Model file for the job. Use its own axes, mm. A direction names the side the tool comes from. Round coordinates to 2 decimals unless told otherwise and drop trailing zeros. Order: outer loops, then holes, each group sorted by start corner. A loop starts at its lowest first (then second) coordinate and runs counter-clockwise, first axis right, second up. Notation, with made-up numbers: M 5.5,-21 L 27.5,-21 A17 ccw 27.5,5 Z; hole C 30,74.25 d5. An arc over 180 degrees is marked long. Return JSON: item names as keys, results as strings. Group by question number.
Item 1: Which spindle directions (+Z, -Z, +X, -X, +Y, -Y) get a long thin tool onto all of the face, cutting with end or side? Do faces 5 (the face through (64, 20, 0.711)), 6 (the face through (51, 17, 0)), 7 (the face through (19, 31, 4.369)). Say none if no direction does.
Item 2: Slice it at A-A on z = 2.3. Write the cut outline in (x, y), then the cut area to 3 significant figures.
Item 3: Probe line 1 along X through (y, z) = (31.5, 3.4); line 2 along Z through (x, y) = (23, 29); line 3 along Y through (x, z) = (10, 3.25). List the from-to ranges inside material, lowest first.
Item 4: Pin check, flat tip, straight feed: pin 1 Ø4.5 at (x, y) = (64, 20.5) entering from -Z. Stop position of the tip, or through.
Item 5: Slice it at B-B on x = 65. Write the cut outline in (y, z), then the cut area to 3 significant figures.
Item 6: Pull direction X, two halves, no side cores. Call faces 1 (the face through (51, 0, 3)), 2 (the face through (18.53, 27.89, 2.15)), 3 (the face through (104.14, 16, 3)), 4 (the face through (61.53, 20.27, 0.35)): pulls with the +X half, pulls with the -X half, needs draft (parallel to the pull), parting line crosses it, or undercut.
Item 7: Slice it at C-C on x = 28.5. Write the cut outline in (y, z), then the cut area to 3 significant figures.
from build123d import *

# Parameters (mm, degrees)
SKETCH1_W           = 104.14
SKETCH1_H           = 33.02
BOSS_EXTRUDE1_DEPTH = 5.334
CAVITY1_DEPTH       = 4.3688
CAVITY1_2_OUTLINE_R = 2.794
CAVITY1_2_DEPTH     = 0.7112


# Read off the part's stored shape, not the designer's step: Cavity1
with BuildPart() as part:
    # Sketch1 → Boss-Extrude1 (new body)
    with BuildSketch(Plane.XY):
        with Locations((52.07, 16.51)):
            Rectangle(SKETCH1_W, SKETCH1_H)
    extrude(amount=BOSS_EXTRUDE1_DEPTH)

    # Cavity1 outline → Cavity1 (cut)
    with BuildSketch(Plane.XY):
        with BuildLine():
            ThreePointArc((7.993160963, 33.02), (18.702187299, 27.889223026), (29.411213634, 33.02))
            Line((29.411213634, 33.02), (7.993160963, 33.02))
        make_face()
    extrude(amount=CAVITY1_DEPTH, mode=Mode.SUBTRACT)

    # Cavity1 2 outline → Cavity1 2 (cut)
    with BuildSketch(Plane.XY):
        with Locations((64.319453414, 20.142181246)):
            Circle(CAVITY1_2_OUTLINE_R)
    extrude(amount=CAVITY1_2_DEPTH, mode=Mode.SUBTRACT)


solid = part.part
Output values:
{
 "1": {"face 5": "-Z", "face 6": "-Z, +X, -X, +Y, -Y", "face 7": "-Z, +Y"},
 "2": {"outline": "M 0,0 L 104.14,0 L 104.14,33.02 L 29.41,33.02 A13.74 cw 7.99,33.02 L 0,33.02 Z", "area": "3,360 mm²"},
 "3": {"line 1": "0 to 9.42, 27.99 to 104.14", "line 2": "4.37 to 5.33", "line 3": "0 to 31"},
 "4": {"pin 1": "z = 0.71"},
 "5": {"outline": "M 0,0 L 17.43,0 L 17.43,0.71 L 22.85,0.71 L 22.85,0 L 33.02,0 L 33.02,5.33 L 0,5.33 Z", "area": "172 mm²"},
 "6": {"face 1": "needs draft", "face 2": "undercut", "face 3": "pulls with the +X half", "face 4": "undercut"},
 "7": {"outline": "M 0,0 L 32,0 L 32,4.37 L 33.02,4.37 L 33.02,5.33 L 0,5.33 Z", "area": "172 mm²"}
}
